Source: CAD feature listing. Evaluate the final solid. Frame: model axes, mm. A direction names the side the tool comes from. Round coordinates to 2 decimals unless told otherwise and drop trailing zeros. Order: outer loops, then holes, each group sorted by start corner. A loop starts at its lowest first (then second) coordinate and runs counter-clockwise, first axis right, second up. Notation, with made-up numbers: (-29, 72) -> (2, 72) arc R23 ccw to (2, 94) -> close; hole circle Ø1 at (51, -25.75). An arc over 180 degrees is marked (long way). Use a Markdown table: item, result. Add a question column.
```python
from build123d import *

# Parameters (mm, degrees)
F0_W     = 20
F0_H     = 20
F0_W_2   = 40
F1_DEPTH = 3
F3_DEPTH = 1


with BuildPart() as f1:
    # F0 (on Front) → F1 (new body)
    with BuildSketch(Plane.XZ):
        with Locations((-20, 0)):
            Rectangle(F0_W, F0_H)
        Polygon((-30, 10), (-10, 10), (-10, 16.5), align=None)
        Polygon((-10, 10), (30, 10), (-10, 16.5), align=None)
        with Locations((10, 0)):
            Rectangle(F0_W_2, F0_H)
        Polygon((-10, -16.5), (30, -10), (-10, -10), align=None)
        Polygon((-10, -16.5), (-10, -10), (-30, -10), align=None)
    extrude(amount=F1_DEPTH)

    # F2 (on face) → F3 (cut)
    with BuildSketch(Plane.XZ.offset(3)):
        Polygon((-10, -16.5), (-10, -13.5), (-27, -8.5), (-27, 8.5), (-10, 13.5), (-10, 16.5), (-30, 10), (-30, -10), align=None)
        Polygon((27, 8.5), (27, -8.5), (-10, -13.5), (-10, -16.5), (30, -10), (30, 10), (-10, 16.5), (-10, 13.5), align=None)
    extrude(amount=-F3_DEPTH, mode=Mode.SUBTRACT)


solid = f1.part
```
1) First-contact query: pin 1 Ø0.5 at (y, z) = (-2.5, -2.5) entering from +X; pin 2 Ø1.5 at (x, y) = (13, -1) entering from +Z. Flat tips, straight axial feed; report the tip coordinate or a pass-through.
2) Section B-B on z = 7. Output: boundary loops of the cut face in (x, y), then the cut area to 3 significant figures.
3) Section C-C on x = -24.5. Output: boundary loops of the cut face in (y, z).
4) Reachability of faces 1 (the flat face through (8.759, -2.507, -10.965)), 2 (the flat face through (-18.381, -2.507, -11.035)), 3 (the flat face through (8.241, -2.507, 11.035)), 4 (the flat face through (-18.619, -2.507, 10.965)) from +Z, -Z, +X, -X, +Y, -Y: full face, straight path, thin tool, end or side. Return the list, or none.
5) Line query: probe 1 along X at (y, z) = (-2.8, 7.5); probe 2 along Y at (x, z) = (-2, 14.5); probe 3 along Z at (x, y) = (-23.5, -0.05). Output: solid intervals per line, ascending. Write a range as from..to.
6) Section A-A on y = -1. Output: boundary loops of the cut face in (x, z).
Conclusion:
| question | item | result |
|---|---|---|
| 1 | pin 1 | stops at x = 27 |
| 1 | pin 2 | stops at z = 12.88 |
| 2 | outline | (-30, -2) -> (-27, -2) -> (-27, -3) -> (27, -3) -> (27, -2) -> (30, -2) -> (30, 0) -> (-30, 0) -> close |
| 2 | area | 174 mm^2 |
| 3 | outline | (-3, -9.24) -> (-2, -9.24) -> (-2, -11.79) -> (0, -11.79) -> (0, 11.79) -> (-2, 11.79) -> (-2, 9.24) -> (-3, 9.24) -> close |
| 4 | face 1 | -Z, +X, -Y |
| 4 | face 2 | -Z, -X, -Y |
| 4 | face 3 | +Z, +X, -Y |
| 4 | face 4 | +Z, -X, -Y |
| 5 | probe 1 | x = -27..27 |
| 5 | probe 2 | y = -2..0 |
| 5 | probe 3 | z = -12.11..12.11 |
| 6 | outline | (-30, -10) -> (-10, -16.5) -> (30, -10) -> (30, 10) -> (-10, 16.5) -> (-30, 10) -> close |
